from build123d import *

# Parameters (mm, degrees)
BOSS_EXTRUDE1_DEPTH = 160
SKETCH2_W           = 76
SKETCH2_H           = 60
BOSS_EXTRUDE2_DEPTH = 60
FILLET1_R           = 30
SKETCH3_R           = 15
CUT_EXTRUDE1_DEPTH  = 201.997512422
RIB1_REACH          = 189.499
SKETCH7_WALL_W      = 497.237426276
SKETCH7_WALL_H      = 12


with BuildPart() as part:
    # Sketch1 → Boss-Extrude1 (new body)
    with BuildSketch(Plane.XY):
        Polygon((-38, 24), (38, 24), (38, 12), (50, 12), (50, 0), (26, 0), (26, 10), (-26, 10), (-26, 0), (-50, 0), (-50, 12), (-38, 12), align=None)
    extrude(amount=-BOSS_EXTRUDE1_DEPTH)

    # Sketch2 → Boss-Extrude2 (add)
    with BuildSketch(Plane(origin=(0, 24, 0), x_dir=(1, 0, 0), z_dir=(0, 1, 0))):
        with Locations((0, 130)):
            Rectangle(SKETCH2_W, SKETCH2_H)
    extrude(amount=BOSS_EXTRUDE2_DEPTH)

    # Fillet1
    fillet1_edges = [part.edges().sort_by_distance(p)[0] for p in [
        (0, 84, -160),
        (0, 84, -100),
    ]]
    fillet(fillet1_edges, radius=FILLET1_R - 0.0001)  # a hair under: the kernel refuses the full size

    # Sketch3 → Cut-Extrude1 (cut, through all)
    with BuildSketch(Plane(origin=(38, 0, 0), x_dir=(0, 0, -1), z_dir=(1, 0, 0))):
        with Locations((130, 54)):
            Circle(SKETCH3_R)
    extrude(amount=-CUT_EXTRUDE1_DEPTH, mode=Mode.SUBTRACT)

    # Sketch7 wall → Rib1 (add, up to next)
    with BuildSketch(Plane(origin=(0, 49.606601718, -54.393398282), x_dir=(0, 0.42592923947, -0.904756477161), z_dir=(0, 0.904756477161, 0.42592923947)), mode=Mode.PRIVATE) as rib1_sk1:
        Rectangle(SKETCH7_WALL_W, SKETCH7_WALL_H)
    rib1_tool1 = extrude(rib1_sk1.sketch, amount=-RIB1_REACH, mode=Mode.PRIVATE) - part.part
    add(rib1_tool1.solids().sort_by_distance((0, 49.606601718, -54.393398282))[0])


solid = part.part
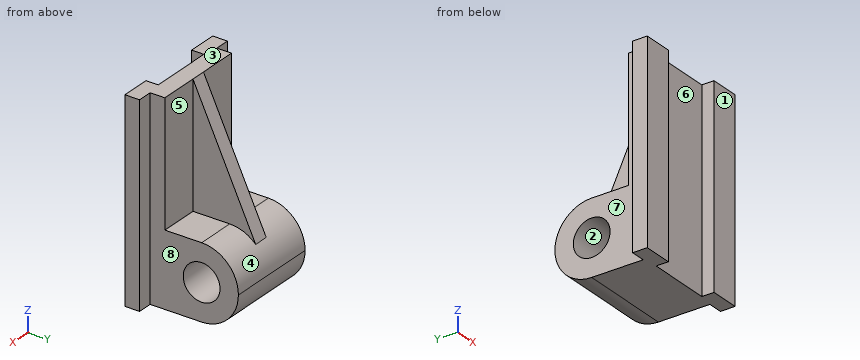
Work out the finished part from the listing and answer in its coordinate system (mm). Face numbers are marked on the shaded views. A direction names the side the tool comes from. Round coordinates to 2 decimals unless told otherwise and drop trailing zeros. Write each loop counter-clockwise with the first axis right and the second up, starting at its lowest first coordinate (ties: lowest second). Pieces come first, ordered by that corner, then holes. Notation, with made-up numbers: (-0.5, 81.25) - (33.5, 81.25) arc R21 cw to (33.5, 107.25) - close; hole circle Ø9 at (82, -26.5). An arc over 180 degrees is marked (long way). Answer in a Markdown table with one row per item. Add a question column.
1. Given pin 1 (16 mm diameter, centred on x = -19, z = -72.5, fed in from +Y); pin 2 (1 mm diameter, centred on x = 18.5, y = 70.5, fed in from -Z); pin 3 (8 mm diameter, centred on x = -1.5, y = 72.5, fed in from +Z), each flat-ended and moving along its own axis, determine where each tip first touches the part or whether it passes through.
2. Find the intervals of material crossed by line 1 along Y through (x, z) = (2.5, -130); line 2 along Y through (x, z) = (46.5, -91.5); line 3 along Z through (x, y) = (-9, 37.5), in increasing order. Write a range as from..to.
3. A cutting plane is placed at D-D, the plane y = 72. Determine the outline of the cut face in (x, z), and give its area (3 significant figures).
4. For the marked faces 4, 5, 6, 7 and 8, determine the directions among +Z, -Z, +X, -X, +Y, -Y from which every point of the face is accessible in a straight line to the end or side of a thin tool.
5. A cutting plane is placed at C-C, the plane z = -120. Determine the outline of the cut face in (x, y).
6. A cutting plane is placed at B-B, the plane y = 49.5. Determine the outline of the cut face in (x, z).
7. The mould has two halves that part along Y. Classify the marked faces 1, 2 and 3: +Y half, -Y half, draft (parallel to the pull), parting line (faces both ways), or undercut.
Worked out:
| question | item | result |
|---|---|---|
| 1 | pin 1 | y = 24 |
| 1 | pin 2 | z = -155.38 |
| 1 | pin 3 | z = -94.53 |
| 2 | line 1 | 10..39, 69..84 |
| 2 | line 2 | 0..12 |
| 2 | line 3 | -160..-100 |
| 3 | outline | (-38, -154) - (38, -154) - (38, -106) - (6, -106) - (6, -101.96) - (-6, -101.96) - (-6, -106) - (-38, -106) - close |
| 3 | area | 3,700 mm^2 |
| 4 | face 4 | +Z, +Y |
| 4 | face 5 | +Z, +X, +Y |
| 4 | face 6 | +Z, -Z, -Y |
| 4 | face 7 | +Z, -Z, -X, +Y |
| 4 | face 8 | +Z, -Z, +X, +Y |
| 5 | outline | (-50, 0) - (-26, 0) - (-26, 10) - (26, 10) - (26, 0) - (50, 0) - (50, 12) - (38, 12) - (38, 42.82) - (-38, 42.82) - (-38, 12) - (-50, 12) - close; (-38, 65.18) - (38, 65.18) - (38, 82.28) - (-38, 82.28) - close |
| 6 | outline | (-38, -160) - (38, -160) - (38, -144.31) - (-38, -144.31) - close; (-38, -115.69) - (38, -115.69) - (38, -100) - (6, -100) - (6, -54.17) - (-6, -54.17) - (-6, -100) - (-38, -100) - close |
| 7 | face 1 | -Y half |
| 7 | face 2 | undercut |
| 7 | face 3 | draft |
